The listing builds one solid part. Answer for the finished solid, in the listing's coordinates (mm). A direction names the side the tool comes from. Coordinates: 2 decimals unless noted, no trailing zeros. Write each loop counter-clockwise with the first axis right and the second up, starting at its lowest first coordinate (ties: lowest second). Pieces come first, ordered by that corner, then holes. Notation, with made-up numbers: M 45.5,69.5 L 76.5,69.5 A29 cw 76.5,105.5 Z; hole C 54.5,17 d4. An arc over 180 degrees is marked long. Write item = value, one per line. Start each with the question number.
```python
from build123d import *

# Parameters (mm, degrees)
ENL_V_START             = 6
ENL_V_MAT_EXTRU_2_DEPTH = 21.343879745


with BuildPart() as part:
    # Esquisse1 → base (revolve)
    with BuildSketch(Plane(origin=(0, 0, 0), x_dir=(0, 0, -1), z_dir=(1, 0, 0)), mode=Mode.PRIVATE) as base_sk:
        with BuildLine():
            Line((0, 1.55), (0, 3))
            Line((0, 3), (-6, 3))
            Line((-6, 3), (-6, 2))
            Line((-6, 2), (-10.45, 2))
            Line((-10.45, 2), (-10.5, 1.9))
            Line((-10.5, 1.9), (-10.55, 2))
            Line((-10.55, 2), (-12.5, 2))
            ThreePointArc((-12.5, 2), (-16.5, 2.5), (-20.5, 2))
            Line((-20.5, 2), (-22.45, 2))
            Line((-22.45, 2), (-22.5, 1.9))
            Line((-22.5, 1.9), (-22.55, 2))
            Line((-22.55, 2), (-24.2, 2))
            Line((-24.2, 2), (-25.4, 1.4))
            ThreePointArc((-25.4, 1.4), (-25.843680391, 0.761577311), (-26, 0))
            Line((-26, 0), (-7, 0))
            Line((-7, 0), (-7, 0.95))
            Line((-7, 0.95), (-6.7, 1.25))
            Line((-6.7, 1.25), (-0.3, 1.25))
            Line((-0.3, 1.25), (0, 1.55))
        make_face()
        with BuildLine():
            Line((-12.92788578, 2), (-12.92788578, 1.9))
            Line((-12.92788578, 1.9), (-20.07211422, 1.9))
            Line((-20.07211422, 1.9), (-20.07211422, 2))
            ThreePointArc((-20.07211422, 2), (-16.5, 2.4), (-12.92788578, 2))
        make_face(mode=Mode.SUBTRACT)
    revolve(base_sk.sketch.rotate(Axis((0, 0, 0), (0, 0, 1)), 90), axis=Axis((0, 0, 0), (0, 0, 1)))

    # Esquisse2 → Enlèv. mat.-Extru.2 (cut, through all)
    with BuildSketch(Plane.XY.offset(ENL_V_START)):
        Polygon((0.3, 2.5), (-0.3, 2.5), (0, 2), align=None)
        Polygon((1.836782357, 1.722274825), (1.285575219, 1.532088886), (1.377155691, 2.107947391), align=None)
        Polygon((2.514113836, 0.138678118), (1.969615506, 0.347296355), (2.409924929, 0.72956277), align=None)
        Polygon((2.015063509, -1.509807621), (1.732050808, -1), (2.315063509, -0.990192379), align=None)
        Polygon((0.573142572, -2.451837595), (0.684040287, -1.879385242), (1.136958145, -2.246625509), align=None)
        Polygon((-1.136958145, -2.246625509), (-0.684040287, -1.879385242), (-0.573142572, -2.451837595), align=None)
        Polygon((-2.315063509, -0.990192379), (-1.732050808, -1), (-2.015063509, -1.509807621), align=None)
        Polygon((-2.409924929, 0.72956277), (-1.969615506, 0.347296355), (-2.514113836, 0.138678118), align=None)
        Polygon((-1.377155691, 2.107947391), (-1.285575219, 1.532088886), (-1.836782357, 1.722274825), align=None)
    extrude(amount=ENL_V_MAT_EXTRU_2_DEPTH, mode=Mode.SUBTRACT)


solid = part.part
```
1. For faces 1 (the face through (-1.812, -0.571, 16.55)), 2 (the face through (1.25, -0.05, 3.46)), 3 (the face through (0, 2, 23)), 4 (the face through (1.3, 1.3, 0)), determine the directions among +Z, -Z, +X, -X, +Y, -Y from which every point of the face is accessible in a straight line to the end or side of a thin tool.
2. The part is cut by section B-B, the plane z = 22. Write down the section's boundary in (x, y), and give its area (3 significant figures).
3. Each of these flat-tipped pins is pushed along its axis until it touches: pin 1 (2 mm diameter, centred on y = -2, z = 22.5, fed in from -X); pin 2 (1.5 mm diameter, centred on x = 1.5, z = 4.5, fed in from +Y); pin 3 (1.8 mm diameter, centred on x = -1.5, y = -0.5, fed in from +Z). Where does it stop, or does it pass through?
4. Straight lines are drawn through the part: L1, parallel to Y at x = 0, z = 3.5; L2, parallel to Z at x = -1.4, y = 1.65; L3, parallel to X at y = 0.2, z = 6.75. For each, find the intervals that lie inside material, in ascending order. Write a range as [from, to].
5. The part is cut by section A-A, the plane z = 14.25. Count the separate pieces of the cut face and the enclosed holes in it, and give its area (3 significant figures).
6. For a pull along Z with two mould halves and no side action, classify faces 5 (the face through (0, 2, 8)), 6 (the face through (0, 0, 7)), 7 (the face through (-2.86, -0.9, 3.04)) as pulls with the +Z half, pulls with the -Z half, needs draft (parallel to the pull), parting line crosses it, or undercut.
Solution:
q1.face_1 = none
q1.face_2 = -Z
q1.face_3 = +Z
q1.face_4 = -Z, +X, -X, +Y, -Y
q2.outline = C 0,0 d4
q2.area = 12.6 mm^2
q3.pin_1 = -1.73
q3.pin_2 = 2.9
q3.pin_3 = 25.88
q4.L1 = [-3, -1.25], [1.25, 3]
q4.L2 = [0, 6]
q4.L3 = [-1.99, -1.18], [1.18, 1.99]
q5.separate_pieces = 10
q5.enclosed_holes = 0
q5.area = 12.5 mm^2
q6.face_5 = undercut
q6.face_6 = pulls with the -Z half
q6.face_7 = needs draft
